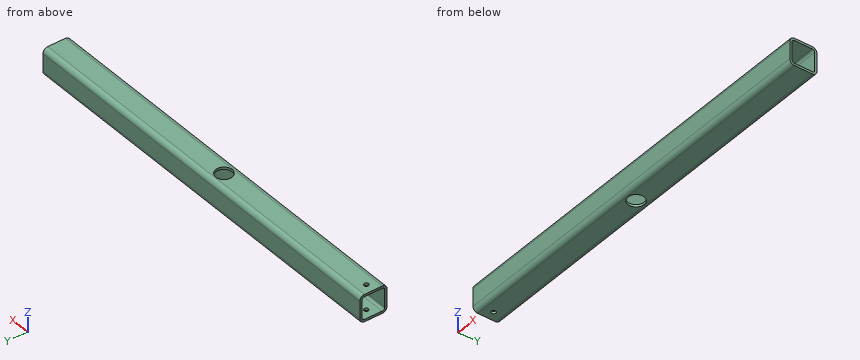
```python
from build123d import *

# Parameters (mm, degrees)
RURA_KWADRATOWA_30_X_30_X_2_6_1_DEPTH = 450
SZKIC2_R                              = 2.5
SZKIC2_R_2                            = 9
WYTNIJ_WYCI_GNI_CIE1_DEPTH            = 228.486263322


with BuildPart() as part:
    # Sketch1 → Rura kwadratowa 30 X 30 X 2.6(1) (new body)
    with BuildSketch(Plane(origin=(-225, 0, 0), x_dir=(0, 0, -1), z_dir=(1, 0, 0))):
        with BuildLine():
            Line((-9.8, -15), (9.8, -15))
            ThreePointArc((9.8, -15), (13.476955262, -13.476955262), (15, -9.8))
            Line((15, -9.8), (15, 9.8))
            ThreePointArc((15, 9.8), (13.476955262, 13.476955262), (9.8, 15))
            Line((9.8, 15), (-9.8, 15))
            ThreePointArc((-9.8, 15), (-13.476955262, 13.476955262), (-15, 9.8))
            Line((-15, 9.8), (-15, -9.8))
            ThreePointArc((-15, -9.8), (-13.476955262, -13.476955262), (-9.8, -15))
        make_face()
        with BuildLine():
            Line((-9.8, -12.4), (9.8, -12.4))
            ThreePointArc((9.8, -12.4), (11.638477631, -11.638477631), (12.4, -9.8))
            Line((12.4, -9.8), (12.4, 9.8))
            ThreePointArc((12.4, 9.8), (11.638477631, 11.638477631), (9.8, 12.4))
            Line((9.8, 12.4), (-9.8, 12.4))
            ThreePointArc((-9.8, 12.4), (-11.638477631, 11.638477631), (-12.4, 9.8))
            Line((-12.4, 9.8), (-12.4, -9.8))
            ThreePointArc((-12.4, -9.8), (-11.638477631, -11.638477631), (-9.8, -12.4))
        make_face(mode=Mode.SUBTRACT)
    extrude(amount=RURA_KWADRATOWA_30_X_30_X_2_6_1_DEPTH)

    # Szkic2 → Wytnij-wyciągnięcie1 (cut, through all)
    with BuildSketch(Plane.XY.offset(15)):
        with Locations((-215, 0)):
            Circle(SZKIC2_R)
        with Locations((-12.73, 0)):
            Circle(SZKIC2_R_2)
    extrude(amount=-WYTNIJ_WYCI_GNI_CIE1_DEPTH, mode=Mode.SUBTRACT)


solid = part.part
```
The listing builds one solid part. Answer for the finished solid, in the listing's coordinates (mm). Coordinates: 2 decimals unless noted, no trailing zeros. Loops run counter-clockwise (first coordinate to the right, second up) from the corner with the lowest first, then second, coordinate; pieces in that order, holes last. Notation, with made-up numbers: (73.5, 84) -> (129.5, 84) arc R24 ccw to (129.5, 103) -> close; hole circle Ø7 at (43.25, 1). An arc over 180 degrees is marked (long way). Return JSON: item names as keys, results as strings. Group by question number.
(1) A cutting plane is placed at B-B on z = 5.75. Write down the section's boundary in (x, y).
(2) Find the intervals of material crossed by probe 1 along Y at (x, z) = (102, -1); probe 2 along Y at (x, z) = (-12.73, 13.7), in increasing order. Write a range as from..to.
(3) A cutting plane is placed at A-A on x = -45. Write down the section's boundary in (y, z), and give its area (3 significant figures).
(4) Given pin 1 Ø1.5 at (x, z) = (33, -12) entering from +Y; pin 2 Ø6.5 at (x, y) = (-215, 0) entering from -Z, each flat-ended and moving along its own axis, determine where each tip first touches the part or whether it passes through.
The answers:
{
 "1": {"outline": "(-225, -15) -> (225, -15) -> (225, -12.4) -> (-225, -12.4) -> close; (-225, 12.4) -> (225, 12.4) -> (225, 15) -> (-225, 15) -> close"},
 "2": {"probe 1": "y = -15..-12.4, 12.4..15", "probe 2": "y = -13.24..-9, 9..13.24"},
 "3": {"outline": "(-15, -9.8) arc R5.2 ccw to (-9.8, -15) -> (9.8, -15) arc R5.2 ccw to (15, -9.8) -> (15, 9.8) arc R5.2 ccw to (9.8, 15) -> (-9.8, 15) arc R5.2 ccw to (-15, 9.8) -> close; hole (-12.4, -9.8) arc R2.6 ccw to (-9.8, -12.4) -> (9.8, -12.4) arc R2.6 ccw to (12.4, -9.8) -> (12.4, 9.8) arc R2.6 ccw to (9.8, 12.4) -> (-9.8, 12.4) arc R2.6 ccw to (-12.4, 9.8) -> close", "area": "268 mm^2"},
 "4": {"pin 1": "stops at y = 14.79", "pin 2": "stops at z = -15"}
}
